Geometry check sheet. Reference: the model listing, model coordinates, mm. A direction names the side the tool comes from. Coordinates: 2 decimals unless noted, no trailing zeros. Write each loop counter-clockwise with the first axis right and the second up, starting at its lowest first coordinate (ties: lowest second). Pieces come first, ordered by that corner, then holes. Notation, with made-up numbers: M 7,78.25 L 65,78.25 A16 ccw 65,108.25 Z; hole C 83.25,-3 d7. An arc over 180 degrees is marked long. Put each result on its own line as item: value. Start each with the question number.
1) Cross-section at A-A on x = 59.69. Record the cut outline in (y, z).
2) Gauge pin test, flat ends, axial feed: pin 1 (1.5 mm diameter, centred on y = 2, z = 22, fed in from -X); pin 2 (1.9 mm diameter, centred on x = 88, y = 3, fed in from -Z); pin 3 (1.8 mm diameter, centred on x = 31.496, y = 3.175, fed in from -Z). Record the tip position at first contact, or that the pin passes through.
3) Cross-section at C-C on x = 50.5. Record the cut outline in (y, z), plus the area to 3 significant figures.
4) Set-up check for faces 1 (the cylindrical face through (84.654, 0.764, -2.946)), 2 (the cylindrical face through (86.885, 3.219, -2.946)), 3 (the flat face through (30, 3, 4.826)): record each of +Z, -Z, +X, -X, +Y, -Y from which the full face is reachable in a straight line by a thin tool's end or side.
5) Mould release check, pull along X, two halves, no side actions. Record for faces 4 (the cylindrical face through (57.5, 3.1, -33.2)), 5 (the flat face through (31, 6.35, 2)), 6 (the cylindrical face through (28.255, 3.131, 16.351)): released by +X, released by -X, zero draft, split by the parting line, or undercut.
6) Scan lines: line 1 along Y through (x, z) = (59.69, 34.3); line 2 along Z through (x, y) = (40, 3); line 3 along X through (y, z) = (5.25, -22.5). Record each from-to range of solid material in increasing order.
7) Cross-section at B-B on z = -9.5. Record the cut outline in (x, y), plus the area to 3 significant figures.
from build123d import *

# Parameters (mm, degrees)
SKETCH1_R                       = 35.433
SKETCH1_R_2                     = 33.274
BOSS_EXTRUDE1_DEPTH             = 6.35
BOSS_EXTRUDE2_START             = 1.016
SKETCH2_R                       = 1
BOSS_EXTRUDE2_DEPTH             = 3.81
BOSS_EXTRUDE3_DEPTH             = 0.00254
BOSS_EXTRUDE3_DEPTH_BACK        = 3.81
BOSS_EXTRUDE3_START             = -1.016
SKETCH3_R                       = 1
CUT_EXTRUDE1_START              = 27.94
SKETCH4_R                       = 1.7526
CUT_EXTRUDE1_DEPTH              = 17.272
CIRPATTERN1_COUNT               = 2
CIRPATTERN1_ANGLE               = 70
CIRPATTERN1_THE_OTHER_WAY_COUNT = 2
CIRPATTERN1_THE_OTHER_WAY_ANGLE = 70
CUT_EXTRUDE2_START              = -42.164
SKETCH5_R                       = 1.7526
CUT_EXTRUDE2_DEPTH              = 42.164
SKETCH6_R                       = 1.905
CUT_EXTRUDE3_DEPTH              = 40.386
SKETCH7_R                       = 1.905
CUT_EXTRUDE4_DEPTH              = 38.1


with BuildPart() as part:
    # Sketch1 → Boss-Extrude1 (new body)
    with BuildSketch(Plane(origin=(0, 0, 0.20701), x_dir=(1, 0, 0), z_dir=(0, 1, 0))):
        with Locations(Location((59.69, 0.20574, 0), (0, 0, 270))):
            Circle(SKETCH1_R)
        with Locations(Location((59.69, 0.20574, 0), (0, 0, 270))):
            Circle(SKETCH1_R_2, mode=Mode.SUBTRACT)
    extrude(amount=BOSS_EXTRUDE1_DEPTH)

    # Sketch2 → Boss-Extrude2 (add)
    with BuildSketch(Plane.XY.offset(BOSS_EXTRUDE2_START)):
        with BuildLine():
            Line((33.02, 6.35), (25.4, 6.35))
            Line((25.4, 6.35), (25.4, 0))
            Line((25.4, 0), (33.02, 0))
            ThreePointArc((33.02, 0), (34.816051224, 0.743948776), (35.56, 2.54))
            Line((35.56, 2.54), (35.56, 3.81))
            ThreePointArc((35.56, 3.81), (34.816051224, 5.606051224), (33.02, 6.35))
        make_face()
        with Locations(Location((31.496, 3.175, 0), (0, 0, 180))):
            Circle(SKETCH2_R, mode=Mode.SUBTRACT)
    extrude(amount=BOSS_EXTRUDE2_DEPTH)

    # Sketch3 → Boss-Extrude3 (add, two sides: drawn at the far end of the back side and taken through both)
    with BuildSketch(Plane.XY.offset(BOSS_EXTRUDE3_START - BOSS_EXTRUDE3_DEPTH_BACK)):
        with BuildLine():
            Line((93.98, 6.35), (86.469496204, 6.35))
            ThreePointArc((86.469496204, 6.35), (84.67344498, 5.606051224), (83.929496204, 3.81))
            Line((83.929496204, 3.81), (83.929496204, 2.54))
            ThreePointArc((83.929496204, 2.54), (84.67344498, 0.743948776), (86.469496204, 0))
            Line((86.469496204, 0), (93.98, 0))
            Line((93.98, 0), (93.98, 6.35))
        make_face()
        with Locations((87.884, 3.175)):
            Circle(SKETCH3_R, mode=Mode.SUBTRACT)
    extrude(amount=BOSS_EXTRUDE3_DEPTH + BOSS_EXTRUDE3_DEPTH_BACK)

    # Sketch4 → Cut-Extrude1 (cut)
    with BuildSketch(Plane.XY.offset(CUT_EXTRUDE1_START)):
        with Locations((59.69, 3.175)):
            Circle(SKETCH4_R)
    cut_extrude1 = extrude(amount=CUT_EXTRUDE1_DEPTH, mode=Mode.SUBTRACT)

    # CirPattern1: Cut-Extrude1 ×2 about axis
    cirpattern1_axis = Axis((59.69, 0, 0.00127), (0, -1, 0))
    for i in range(1, CIRPATTERN1_COUNT):
        add(cut_extrude1.rotate(cirpattern1_axis, i * CIRPATTERN1_ANGLE / (CIRPATTERN1_COUNT - 1)), mode=Mode.SUBTRACT)

    # CirPattern1 the other way: Cut-Extrude1 ×2 about axis
    cirpattern1_the_other_way_axis = Axis((59.69, 0, 0.00127), (0, 1, 0))
    for i in range(1, CIRPATTERN1_THE_OTHER_WAY_COUNT):
        add(cut_extrude1.rotate(cirpattern1_the_other_way_axis, i * CIRPATTERN1_THE_OTHER_WAY_ANGLE / (CIRPATTERN1_THE_OTHER_WAY_COUNT - 1)), mode=Mode.SUBTRACT)

    # Sketch5 → Cut-Extrude2 (cut)
    with BuildSketch(Plane.XY.offset(CUT_EXTRUDE2_START)):
        with Locations((59.69, 3.175)):
            Circle(SKETCH5_R)
    extrude(amount=CUT_EXTRUDE2_DEPTH, mode=Mode.SUBTRACT)

    # Sketch6 → Cut-Extrude3 (cut)
    with BuildSketch(Plane.XY.offset(-1.01346)):
        with Locations(Location((87.884, 3.175, 0), (0, 0, 180))):
            Circle(SKETCH6_R)
    extrude(amount=CUT_EXTRUDE3_DEPTH, mode=Mode.SUBTRACT)

    # Sketch7 → Cut-Extrude4 (cut)
    with BuildSketch(Plane(origin=(0, 0, 1.016), x_dir=(-1, 0, 0), z_dir=(0, 0, -1))):
        with Locations(Location((-31.496, 3.175, 0), (0, 0, 180))):
            Circle(SKETCH7_R)
    extrude(amount=CUT_EXTRUDE4_DEPTH, mode=Mode.SUBTRACT)


solid = part.part
Answer key:
1. outline: M 0,-35.43 L 1.42,-35.43 L 1.42,-33.27 L 0,-33.27 Z; M 0,33.28 L 1.42,33.28 L 1.42,35.43 L 0,35.43 Z; M 4.93,-35.43 L 6.35,-35.43 L 6.35,-33.27 L 4.93,-33.27 Z; M 4.93,33.28 L 6.35,33.28 L 6.35,35.43 L 4.93,35.43 Z
2. pin 1: stops at x = 31.34
2. pin 2: stops at z = -22.51
2. pin 3: stops at z = 16.15
3. outline: M 0,-34.22 L 6.35,-34.22 L 6.35,-31.98 L 0,-31.98 Z; M 0,31.98 L 6.35,31.98 L 6.35,34.22 L 0,34.22 Z
3. area: 28.5 mm²
4. face 1: -Y
4. face 2: +Z
4. face 3: +Y, -Y
5. face 4: undercut
5. face 5: zero draft
5. face 6: split by the parting line
6. line 1: y = 0 to 1.42, 4.93 to 6.35
6. line 2: z = -29.46 to -26.82, 26.82 to 29.46
6. line 3: x = 32.32 to 35.18, 84.2 to 87.06
7. outline: M 25.55,0 L 27.8,0 L 27.8,6.35 L 25.55,6.35 Z; M 91.58,0 L 93.83,0 L 93.83,6.35 L 91.58,6.35 Z
7. area: 28.5 mm²
